```python
from build123d import *

# Parameters (mm, degrees)
F0_R     = 12.7
F1_DEPTH = 508
F2_DEPTH = 127
F3_DEPTH = 50.8


with BuildPart() as f1:
    # F0 (on Front) → F1 (new body)
    with BuildSketch(Plane.XZ):
        with Locations((0, -3.2373953145)):
            Circle(F0_R)
    extrude(amount=F1_DEPTH)

    # F2 (cut): a face of the model
    f2_faces = [f1.faces().sort_by_distance(p)[0] for p in [
        (0, -508, -3.2373953145),
    ]]
    extrude(f2_faces, amount=-F2_DEPTH, mode=Mode.SUBTRACT)

    # F3 (cut): a face of the model
    f3_faces = [f1.faces().sort_by_distance(p)[0] for p in [
        (0, -381, -3.2373953145),
    ]]
    extrude(f3_faces, amount=-F3_DEPTH, mode=Mode.SUBTRACT)


solid = f1.part
```
Work out the finished part from the listing and answer in its coordinate system (mm). Coordinates: 2 decimals unless noted, no trailing zeros. Loops run counter-clockwise (first coordinate to the right, second up) from the corner with the lowest first, then second, coordinate; pieces in that order, holes last. Notation, with made-up numbers: (52, -11) - (79, -11) arc R20 ccw to (79, 11) - close; hole circle Ø11 at (49, 7.25). An arc over 180 degrees is marked (long way). Use a Markdown table: item, result.
Item 1: Find section B-B, the plane x = 5. Determine the outline of the cut face in (y, z).
Evaluation:
| item | result |
|---|---|
| outline | (-330.2, -14.91) - (0, -14.91) - (0, 8.44) - (-330.2, 8.44) - close |
Item 2: Find section A-A, the plane z = 5.5. Determine the outline of the cut face in (x, y).
Evaluation:
| item | result |
|---|---|
| outline | (-9.22, -330.2) - (9.22, -330.2) - (9.22, 0) - (-9.22, 0) - close |
Item 3: Given pin 1 Ø8 at (y, z) = (-109, 2) entering from -X; pin 2 Ø5 at (x, y) = (5, -188.5) entering from -Z; pin 3 Ø10 at (y, z) = (-250, -9) entering from -X, each flat-ended and moving along its own axis, determine where each tip first touches the part or whether it passes through.
Evaluation:
| item | result |
|---|---|
| pin 1 | stops at x = -12.64 |
| pin 2 | stops at z = -15.69 |
| pin 3 | stops at x = -12.68 |
Item 4: Consider probe 1 along Z at (x, y) = (-1.25, -257); probe 2 along X at (y, z) = (-247, -2.25); probe 3 along Z at (x, y) = (0.25, -191). Determine where each line is inside the solid, lowest interval first. Write a range as from..to.
Evaluation:
| item | result |
|---|---|
| probe 1 | z = -15.88..9.4 |
| probe 2 | x = -12.66..12.66 |
| probe 3 | z = -15.93..9.46 |
Item 5: Find section C-C, the plane y = -254. Determine the outline of the cut face in (x, z).
Evaluation:
| item | result |
|---|---|
| outline | circle Ø25.4 at (0, -3.24) |
